```python
from build123d import *

# Parameters (mm, degrees)
BOSS_EXTRUDE1_DEPTH = 19.05
SKETCH4_R           = 1.6383
CUT_EXTRUDE1_DEPTH  = 4.175
SKETCH5_R           = 2.54
CUT_EXTRUDE2_DEPTH  = 6.953125


with BuildPart() as part:
    # Sketch1 → Boss-Extrude1 (new body)
    with BuildSketch(Plane(origin=(0, 0, 0), x_dir=(1, 0, 0), z_dir=(0, 1, 0))):
        with BuildLine():
            Line((0.396875, 9.516728179), (0.396875, 4.231428864))
            ThreePointArc((0.396875, 4.231428864), (4.25, 0), (0.396875, -4.231428864))
            Line((0.396875, -4.231428864), (0.396875, -9.516728179))
            ThreePointArc((0.396875, -9.516728179), (9.525, 0), (0.396875, 9.516728179))
        make_face()
    extrude(amount=BOSS_EXTRUDE1_DEPTH)

    # Sketch4 → Cut-Extrude1 (cut, through all)
    with BuildSketch(Plane(origin=(3.571875, 0, 0), x_dir=(0, 0, -1), z_dir=(1, 0, 0))):
        with Locations((-6.874078522, 9.525)):
            Circle(SKETCH4_R)
    cut_extrude1 = extrude(amount=-CUT_EXTRUDE1_DEPTH, mode=Mode.SUBTRACT)

    # Sketch5 → Cut-Extrude2 (cut, through all)
    with BuildSketch(Plane(origin=(3.571875, 0, 0), x_dir=(0, 0, -1), z_dir=(1, 0, 0))):
        with Locations((-6.874078522, 9.525)):
            Circle(SKETCH5_R)
    cut_extrude2 = extrude(amount=CUT_EXTRUDE2_DEPTH, mode=Mode.SUBTRACT)

    # Mirror1: Cut-Extrude1, Cut-Extrude2 across plane
    add(cut_extrude1.mirror(Plane.XY), mode=Mode.SUBTRACT)
    add(cut_extrude2.mirror(Plane.XY), mode=Mode.SUBTRACT)


solid = part.part
```
The model under review builds one solid part; all positions refer to its coordinate system, in mm. A direction names the side the tool comes from. Round coordinates to 2 decimals unless told otherwise and drop trailing zeros. Write each loop counter-clockwise with the first axis right and the second up, starting at its lowest first coordinate (ties: lowest second). Pieces come first, ordered by that corner, then holes. Notation, with made-up numbers: (82, -15) - (110, -15) arc R10 ccw to (110, -9) - close; hole circle Ø11 at (24.5, -31.5). An arc over 180 degrees is marked (long way). Use one line per item in the form item = value.
Q1. Consider section B-B (z = -6). State the section outline as (x, y) points.
Answer key:
outline = (0.4, 0) - (7.4, 0) - (7.4, 7.14) - (3.57, 7.14) - (3.57, 8.14) - (0.4, 8.14) - close; (0.4, 10.91) - (3.57, 10.91) - (3.57, 11.91) - (7.4, 11.91) - (7.4, 19.05) - (0.4, 19.05) - close
Q2. Consider section D-D (y = 4.5). State the section outline as (x, z) points (3 decimals).
Answer key:
outline = (0.397, -9.517) arc R9.525 ccw to (0.397, 9.517) - (0.397, 4.231) arc R4.25 cw to (0.397, -4.231) - close
Q3. Insertion check: pin 1 Ø5 at (y, z) = (9, 7) entering from +X; pin 2 Ø1.3 at (y, z) = (10.5, -6) entering from +X; pin 3 Ø4 at (x, y) = (4.5, 10) entering from -Z. Each pin has a flat end and moves straight along its axis. Give the tip position at first contact, or say it passes through.
Answer key:
pin_1 = 8.37
pin_2 = 3.57
pin_3 = -9.19
Q4. Draft analysis for pull direction Y (two halves, no side actions). For faces 3 (the flat face through (0.397, 9, -5)), 4 (the flat face through (5, 19.05, 0)), 5 (the flat face through (3.572, 10, -5)), state which applies: +Y half, -Y half, draft (parallel to the pull), parting line (faces both ways), or undercut.
Answer key:
face_3 = draft
face_4 = +Y half
face_5 = undercut
Q5. Consider section A-A (x = 2.5). State the section outline as (y, z) points (3 decimals).
Answer key:
outline = (0, -9.191) - (19.05, -9.191) - (19.05, -3.437) - (0, -3.437) - close; (0, 3.437) - (19.05, 3.437) - (19.05, 9.191) - (0, 9.191) - close; hole circle Ø3.277 at (9.525, -6.874); hole circle Ø3.277 at (9.525, 6.874)
Q6. Consider section C-C (x = 4). State the section outline as (y, z) points (3 decimals).
Answer key:
outline = (0, -8.644) - (7.704, -8.644) arc R2.54 cw (long way) to (11.346, -8.644) - (19.05, -8.644) - (19.05, -1.436) - (0, -1.436) - close; (0, 1.436) - (19.05, 1.436) - (19.05, 8.644) - (11.346, 8.644) arc R2.54 cw (long way) to (7.704, 8.644) - (0, 8.644) - close
Q7. Tool access review of faces 1 (the cylindrical face through (5.447, 9.438, 4.336)), 2 (the cylindrical face through (9.523, 9.392, 0.204)): name each direction out of +Z, -Z, +X, -X, +Y, -Y from which nothing blocks a thin tool from reaching the whole face with its end or side.
Answer key:
face_1 = +X
face_2 = +X, +Y, -Y
Q8. For line 1 (Y direction, x = 5, z = 6); line 2 (Y direction, x = 5, z = -6.5); line 3 (X direction, y = 10, z = 5.25), list the stretches that pass through material, from the lowest coordinate up. Write a range as [from, to].
Answer key:
line_1 = [0, 7.14], [11.91, 19.05]
line_2 = [0, 7.01], [12.04, 19.05]
line_3 = [0.4, 3.57]
